from build123d import *

# Parameters (mm, degrees)
F0_W     = 40
F0_H     = 30
F0_R     = 1.55
F0_R_2   = 3
F1_DEPTH = 3


with BuildPart() as f1:
    # F0 (on Front) → F1 (new body)
    with BuildSketch(Plane.XZ):
        Rectangle(F0_W, F0_H)
        with Locations((-15, -10)):
            Circle(F0_R, mode=Mode.SUBTRACT)
        with Locations((15, -10)):
            Circle(F0_R, mode=Mode.SUBTRACT)
        with Locations((-15, 10)):
            Circle(F0_R, mode=Mode.SUBTRACT)
        with Locations((0, 5)):
            Circle(F0_R_2, mode=Mode.SUBTRACT)
        with Locations((15, 10)):
            Circle(F0_R, mode=Mode.SUBTRACT)
    extrude(amount=F1_DEPTH)


solid = f1.part
Verification items for the finished model (mm, model axes). Coordinates: 2 decimals unless noted, no trailing zeros. Write each loop counter-clockwise with the first axis right and the second up, starting at its lowest first coordinate (ties: lowest second). Pieces come first, ordered by that corner, then holes. Notation, with made-up numbers: (77, -3.75) - (133, -3.75) arc R33 ccw to (133, 28.25) - close; hole circle Ø3 at (87.25, 28.25). An arc over 180 degrees is marked (long way). Answer as a JSON object with one key per item and string values.
(1) Thickness scan on line 1 along Z through (x, y) = (15, -1.3); line 2 along Z through (x, y) = (14, -0.65); line 3 along Z through (x, y) = (2.5, -0.8). Record the ranges inside material, lowest first.
Report:
{"line 1": "-15 to -11.55, -8.45 to 8.45, 11.55 to 15", "line 2": "-15 to -11.18, -8.82 to 8.82, 11.18 to 15", "line 3": "-15 to 3.34, 6.66 to 15"}
(2) Mould release check, pull along Z, two halves, no side actions. Record for faces 1 (the cylindrical face through (13.45, -1.48, 10.07)), 2 (the flat face through (0, 0, 0)), 3 (the flat face through (0, -1, -15)): pulls with the +Z half, pulls with the -Z half, needs draft (parallel to the pull), parting line crosses it, or undercut.
Report:
{"face 1": "undercut", "face 2": "needs draft", "face 3": "pulls with the -Z half"}
(3) Cross-section at A-A on z = 10. Record the cut outline in (x, y), plus the area to 3 significant figures.
Report:
{"outline": "(-20, -3) - (-16.55, -3) - (-16.55, 0) - (-20, 0) - close; (-13.45, -3) - (13.45, -3) - (13.45, 0) - (-13.45, 0) - close; (16.55, -3) - (20, -3) - (20, 0) - (16.55, 0) - close", "area": "101 mm^2"}
(4) Cross-section at B-B on x = 0. Record the cut outline in (y, z).
Report:
{"outline": "(-3, -15) - (0, -15) - (0, 2) - (-3, 2) - close; (-3, 8) - (0, 8) - (0, 15) - (-3, 15) - close"}
(5) Cross-section at C-C on x = -15. Record the cut outline in (y, z).
Report:
{"outline": "(-3, -15) - (0, -15) - (0, -11.55) - (-3, -11.55) - close; (-3, -8.45) - (0, -8.45) - (0, 8.45) - (-3, 8.45) - close; (-3, 11.55) - (0, 11.55) - (0, 15) - (-3, 15) - close"}
(6) Cross-section at D-D on y = -1.4. Record the cut outline in (x, z).
Report:
{"outline": "(-20, -15) - (20, -15) - (20, 15) - (-20, 15) - close; hole circle Ø3.1 at (-15, -10); hole circle Ø3.1 at (-15, 10); hole circle Ø6 at (0, 5); hole circle Ø3.1 at (15, -10); hole circle Ø3.1 at (15, 10)"}
